Source: CAD feature listing. Evaluate the final solid. Frame: model axes, mm. A direction names the side the tool comes from. Give positions to 0.01 mm unless a question says otherwise; leave off trailing zeros. Order: outer loops, then holes, each group sorted by start corner. A loop starts at its lowest first (then second) coordinate and runs counter-clockwise, first axis right, second up.
from build123d import *

# Parameters (mm, degrees)
BOSS_EXTRUDE1_DEPTH = 1.5
SKETCH1_4_W         = 11
SKETCH1_4_H         = 2
BOSS_EXTRUDE2_DEPTH = 1


with BuildPart() as part:
    # Sketch1 → Boss-Extrude1 (new, symmetric)
    with BuildSketch(Plane.XY):
        Polygon((-28.5, -6), (-39.5, -6), (-39.5, -9), (-42, -11.5), (-42, -20.5), (-36, -20.5), (-24.008925726, -8.508925726), (-21.5, -6), align=None)
    extrude(amount=BOSS_EXTRUDE1_DEPTH, both=True)

    # Sketch1<4> → Boss-Extrude2 (add, symmetric)
    with BuildSketch(Plane.XY):
        with Locations((-34, -5)):
            Rectangle(SKETCH1_4_W, SKETCH1_4_H)
    extrude(amount=BOSS_EXTRUDE2_DEPTH, both=True)


solid = part.part
1) Section query B-B on x = -33.25. Output: boundary loops of the cut face in (y, z), and give its area (4 significant figures).
Checks:
outline: (-17.75, -1.5) - (-6, -1.5) - (-6, -1) - (-4, -1) - (-4, 1) - (-6, 1) - (-6, 1.5) - (-17.75, 1.5) - close
area: 39.25 mm2
2) Ray query, L1, parallel to Y at x = -27, z = -0.4; L2, parallel to Z at x = -37.5, y = -4.75; L3, parallel to Y at x = -37, z = 1.05. Return the intervals inside material, ascending.
Checks:
L1: y = -11.5 to -6
L2: z = -1 to 1
L3: y = -20.5 to -6
3) Section query C-C on y = -12. Output: boundary loops of the cut face in (x, z).
Checks:
outline: (-42, -1.5) - (-27.5, -1.5) - (-27.5, 1.5) - (-42, 1.5) - close
4) Section query A-A on z = 0.1. Output: boundary loops of the cut face in (x, y), and give its area (4 significant figures).
Checks:
outline: (-42, -20.5) - (-36, -20.5) - (-21.5, -6) - (-28.5, -6) - (-28.5, -4) - (-39.5, -4) - (-39.5, -9) - (-42, -11.5) - close
area: 203.5 mm2
5) Reachability of faces 4 (the face through (-39.5, -6, 0)), 5 (the face through (-28.5, -5, 0)), 6 (the face through (-34, -4, 0)) from +Z, -Z, +X, -X, +Y, -Y: full face, straight path, thin tool, end or side. Return the list, or none.
Checks:
face 4: +Z, -Z, -X, +Y
face 5: +Z, -Z, +X, +Y
face 6: +Z, -Z, +X, -X, +Y
6) Pull-direction query (Z, two-part tool) for faces 1 (the face through (-42, -16, 0)), 2 (the face through (-34, -5, 1)), 3 (the face through (-34, -5, -1)); classes: +Z half, -Z half, draft (parallel to the pull), parting line (faces both ways), or undercut.
Checks:
face 1: draft
face 2: +Z half
face 3: -Z half
7) First-contact query: pin 1 Ø1 at (x, z) = (-31.5, 0) entering from -Y; pin 2 Ø1 at (x, y) = (-34.5, -5) entering from +Z; pin 3 Ø1 at (y, z) = (-5, 0.5) entering from +X. Flat tips, straight axial feed; report the tip coordinate or a pass-through.
Checks:
pin 1: stops at y = -16.5
pin 2: stops at z = 1
pin 3: stops at x = -28.5
8) Section query D-D on x = -23. Output: boundary loops of the cut face in (y, z), and give its area (3 significant figures).
Checks:
outline: (-7.5, -1.5) - (-6, -1.5) - (-6, 1.5) - (-7.5, 1.5) - close
area: 4.50 mm2
